Geometry: final body of the model. Coordinates: model frame, mm. A direction names the side the tool comes from. Round coordinates to 2 decimals unless told otherwise and drop trailing zeros. Write each loop counter-clockwise with the first axis right and the second up, starting at its lowest first coordinate (ties: lowest second). Pieces come first, ordered by that corner, then holes. Notation, with made-up numbers: (76, -15.5) -> (114, -15.5) arc R16 cw to (114, -6.5) -> close; hole circle Ø7 at (81, 78). An arc over 180 degrees is marked (long way). Use one line per item in the form item = value. Start each with the question number.
1. Cut plane B-B, the plane x = 102.5. Return the cut outline in (y, z).
2. Pin query (flat end, axial travel): pin 1 Ø1 at (x, z) = (229, 11.5) entering from +Y; pin 2 Ø5 at (x, z) = (235, 2.5) entering from -Y. Return the tip coordinate at first contact, or that it passes through.
3. Draft query along X for faces 3 (the face through (99, -89, 8)), 4 (the face through (97, -6, 0)). Return one class per face: pulls with the +X half, pulls with the -X half, needs draft (parallel to the pull), parting line crosses it, or undercut.
4. Line query: L1, parallel to X at y = -61.5, z = 6; L2, parallel to Y at x = 107, z = 1.75; L3, parallel to Y at x = 137, z = 8.5. Output: solid intervals per line, ascending.
5. Cut plane C-C, the plane z = 12.25. Return the cut outline in (x, y).
6. Cut plane A-A, the plane y = -67.5. Return the cut outline in (x, z).
7. Reachability of faces 1 (the face through (98, -9, 8)), 2 (the face through (97, -6, 15)) from +Z, -Z, +X, -X, +Y, -Y: full face, straight path, thin tool, end or side. Return the list, or none.
Autodesk Fusion 360 part; units mm, degrees
sketch "Sketch1" plane through (0, 0, 0) normal (0, 0, 1) x (1, 0, 0)
  line L0 (-100, 50) -> (300, 50)
  line L1 (300, 50) -> (300, -150)
  line L2 (300, -150) -> (-100, -150)
  line L3 (-100, -150) -> (-100, 50)
  dimension "d1" = 200
extrude "Extrude1" add sketch "Sketch1" along normal blind 15
ref_plane "WorkPlane1" through (100, -50, 15) normal (0, 0, 1) x (1, 0, 0)
sketch "Sketch2" plane through (0, 0, 15) normal (0, 0, 1) x (1, 0, 0)
  line L0 (60.5, -9) -> (136.5, -9)
  line L1 (139, -11.5) -> (139, -86.5)
  line L2 (136.5, -89) -> (60.5, -89)
  line L3 (58, -86.5) -> (58, -11.5)
  arc A0 (58, -86.5) -> (60.5, -89) centre (60.5, -86.5) ccw
  arc A1 (136.5, -89) -> (139, -86.5) centre (136.5, -86.5) ccw
  arc A2 (139, -11.5) -> (136.5, -9) centre (136.5, -11.5) ccw
  arc A3 (60.5, -9) -> (58, -11.5) centre (60.5, -11.5) ccw
  dimension "d6" = 2.5
extrude "Extrude2" cut sketch "Sketch2" against normal blind 70
fillet "Fillet1" radius 5 1 edges at (100, 50, 15)
fillet "Fillet2" radius 5 1 edges at (100, -150, 15)
fillet "Fillet3" radius 5 5 edges at (300, -150, 5) (300, -148.5355, 13.5355) (300, -50, 15) (300, 48.5355, 13.5355) (300, 50, 5)
fillet "Fillet4" radius 5 5 edges at (97.5, 50, 0) (298.5355, 48.5355, 0) (300, -50, 0) (298.5355, -148.5355, 0) (97.5, -150, 0)
fillet "Fillet5" radius 5 8 edges at (-100, -150, 7.5) (-100, -148.5355, 1.4645) (-100, -50, 0) (-100, 48.5355, 1.4645) (-100, 50, 7.5) (-100, 48.5355, 13.5355) (-100, -50, 15) (-100, -148.5355, 13.5355)
Outcome:
q1.outline = (-150, 5) arc R5 ccw to (-145, 0) -> (-89, 0) -> (-89, 15) -> (-145, 15) arc R5 ccw to (-150, 10) -> close; (-9, 0) -> (45, 0) arc R5 ccw to (50, 5) -> (50, 10) arc R5 ccw to (45, 15) -> (-9, 15) -> close
q2.pin_1 = 49.9
q2.pin_2 = -150
q3.face_3 = undercut
q3.face_4 = needs draft
q4.L1 = -100 to 58, 139 to 300
q4.L2 = -148.8 to -89, -9 to 48.8
q4.L3 = -150 to -88.95, -9.05 to 50
q5.outline = (-99.47, -145) arc R4.47 ccw to (-95, -149.47) -> (295, -149.47) arc R4.47 ccw to (299.47, -145) -> (299.47, 45) arc R4.47 ccw to (295, 49.47) -> (-95, 49.47) arc R4.47 ccw to (-99.47, 45) -> close; hole (58, -86.5) arc R2.5 ccw to (60.5, -89) -> (136.5, -89) arc R2.5 ccw to (139, -86.5) -> (139, -11.5) arc R2.5 ccw to (136.5, -9) -> (60.5, -9) arc R2.5 ccw to (58, -11.5) -> close
q6.outline = (-100, 5) arc R5 ccw to (-95, 0) -> (58, 0) -> (58, 15) -> (-95, 15) arc R5 ccw to (-100, 10) -> close; (139, 0) -> (295, 0) arc R5 ccw to (300, 5) -> (300, 10) arc R5 ccw to (295, 15) -> (139, 15) -> close
q7.face_1 = +Z, -Z
q7.face_2 = +Z, +X, -X, +Y, -Y
